```python
from build123d import *

# Parameters (mm, degrees)
FILLET1_R                    = 1.5
CUT_EXTRUDE1_START           = -35
CUT_EXTRUDE1_DEPTH           = 35
FILLET2_R                    = 2
CIRPATTERN1_COUNT            = 6
FILLET2_OF_CIRPATTERN1_R     = 2
FILLET3_R                    = 5
CHAMFER1_SIZE                = 2
CHAMFER3_SIZE                = 1
CUT_EXTRUDE2_REACH           = 152.223
SKETCH3_W                    = 12
SKETCH3_H                    = 35
CHAMFER4_SIZE                = 0.5
CIRPATTERN2_COUNT            = 6
CHAMFER4_OF_CIRPATTERN2_SIZE = 0.5


with BuildPart() as part:
    # Sketch1 → Revolve1 (revolve)
    with BuildSketch(Plane.XY):
        Polygon((20, 80), (30, 80), (30, 50), (77.5, 50), (77.5, 0), (63, 0), (63, 35), (70, 35), (70, 40), (25, 40), (25, 45), (20, 45), align=None)
    revolve(axis=Axis((0, -1292.390356755, 0), (0, 1, 0)))

    # Fillet1
    fillet1_edges = [part.edges().sort_by_distance(p)[0] for p in [
        (-70, 40, 0),
    ]]
    fillet(fillet1_edges, radius=FILLET1_R)

    # Sketch2 → Cut-Extrude1 (cut)
    with BuildSketch(Plane.XZ.offset(CUT_EXTRUDE1_START)):
        with BuildLine():
            Line((-6.125, 68.8), (6.125, 68.8))
            Line((6.125, 68.8), (6.125, 62.701550021))
            ThreePointArc((6.125, 62.701550021), (0, 63), (-6.125, 62.701550021))
            Line((-6.125, 62.701550021), (-6.125, 68.8))
        make_face()
    cut_extrude1 = extrude(amount=CUT_EXTRUDE1_DEPTH, mode=Mode.SUBTRACT)

    # Fillet2
    fillet2_edges = [part.edges().sort_by_distance(p)[0] for p in [
        (6.125, 17.5, 62.701550021),
        (-6.125, 17.5, 62.701550021),
    ]]
    fillet(fillet2_edges, radius=FILLET2_R)

    # CirPattern1: Cut-Extrude1 ×6 about axis
    cirpattern1_axis = Axis((0, 0, 0), (0, 1, 0))
    for i in range(1, CIRPATTERN1_COUNT):
        add(cut_extrude1.rotate(cirpattern1_axis, i * 360 / CIRPATTERN1_COUNT), mode=Mode.SUBTRACT)

    # Fillet2 of CirPattern1
    fillet2_of_cirpattern1_edges = [part.edges().sort_by_distance(p)[0] for p in [
        (57.363635175, 17.5, 26.046369412),
        (51.238635175, 17.5, 36.655180609),
        (51.238635175, 17.5, -36.655180609),
        (57.363635175, 17.5, -26.046369412),
        (-6.125, 17.5, -62.701550021),
        (6.125, 17.5, -62.701550021),
        (-57.363635175, 17.5, -26.046369412),
        (-51.238635175, 17.5, -36.655180609),
        (-51.238635175, 17.5, 36.655180609),
        (-57.363635175, 17.5, 26.046369412),
    ]]
    fillet(fillet2_of_cirpattern1_edges, radius=FILLET2_OF_CIRPATTERN1_R)

    # Fillet3
    fillet3_edges = [part.edges().sort_by_distance(p)[0] for p in [
        (-30, 50, 0),
    ]]
    fillet(fillet3_edges, radius=FILLET3_R)

    # Chamfer1
    chamfer1_edges = [part.edges().sort_by_distance(p)[0] for p in [
        (-77.5, 50, 0),
        (-30, 80, 0),
        (-20, 80, 0),
    ]]
    chamfer(chamfer1_edges, length=CHAMFER1_SIZE)

    # Chamfer3
    chamfer3_edges = [part.edges().sort_by_distance(p)[0] for p in [
        (-25, 40, 0),
        (-20, 45, 0),
    ]]
    chamfer(chamfer3_edges, length=CHAMFER3_SIZE)

    # Sketch3 → Cut-Extrude2 (cut, up to next)
    with BuildSketch(Plane(origin=(23.3, 0, 0), x_dir=(0, 0, -1), z_dir=(1, 0, 0)), mode=Mode.PRIVATE) as cut_extrude2_sk1:
        with Locations((0, 62.5)):
            Rectangle(SKETCH3_W, SKETCH3_H)
    cut_extrude2_tool1 = extrude(cut_extrude2_sk1.sketch, amount=-CUT_EXTRUDE2_REACH, mode=Mode.PRIVATE) & part.part
    add(cut_extrude2_tool1.solids().sort_by_distance((23.3, 62.5, 0))[0], mode=Mode.SUBTRACT)

    # Sketch6 → Cut-Revolve1 (revolve, cut)
    with BuildSketch(Plane.XY, mode=Mode.PRIVATE) as cut_revolve1_sk:
        Polygon((-67.75, 0), (-67.75, 10), (-70.25, 11.443375673), (-70.25, 0), align=None)
    cut_revolve1 = revolve(cut_revolve1_sk.sketch.rotate(Axis((-70.25, -967.908056453, 0), (0, 1, 0)), 90), axis=Axis((-70.25, -967.908056453, 0), (0, 1, 0)), mode=Mode.SUBTRACT)

    # Chamfer4
    chamfer4_edges = [part.edges().sort_by_distance(p)[0] for p in [
        (-70.25, 0, 2.5),
    ]]
    chamfer(chamfer4_edges, length=CHAMFER4_SIZE)

    # CirPattern2: Cut-Revolve1 ×6 about axis
    cirpattern2_axis = Axis((0, 0, 0), (0, 1, 0))
    for i in range(1, CIRPATTERN2_COUNT):
        add(cut_revolve1.rotate(cirpattern2_axis, i * 360 / CIRPATTERN2_COUNT), mode=Mode.SUBTRACT)

    # Chamfer4 of CirPattern2
    chamfer4_of_cirpattern2_edges = [part.edges().sort_by_distance(p)[0] for p in [
        (-32.959936491, 0, 62.088284616),
        (37.290063509, 0, 59.588284616),
        (70.25, 0, -2.5),
        (32.959936491, 0, -62.088284616),
        (-37.290063509, 0, -59.588284616),
    ]]
    chamfer(chamfer4_of_cirpattern2_edges, length=CHAMFER4_OF_CIRPATTERN2_SIZE)


solid = part.part
```
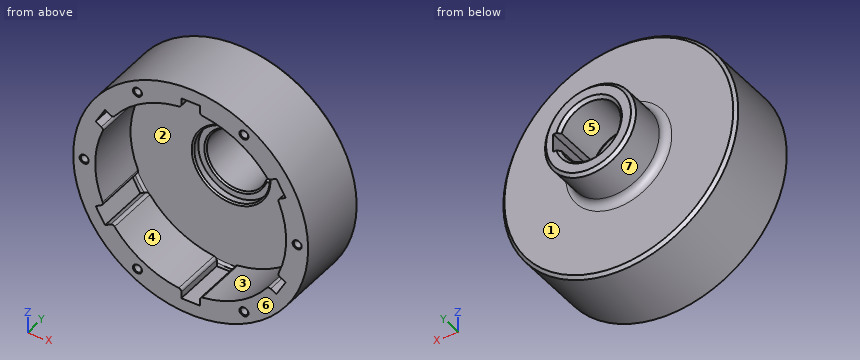
The model under review builds one solid part; all positions refer to its coordinate system, in mm. Face numbers are marked on the shaded views. A direction names the side the tool comes from. Round coordinates to 2 decimals unless told otherwise and drop trailing zeros. Use CSV: the item, a comma, the result in double quotes.
Q1. For pin 1 Ø8 at (x, z) = (-5.5, -49.5) entering from +Y; pin 2 Ø3.5 at (x, y) = (22, 59.5) entering from -Z; pin 3 Ø4.5 at (x, z) = (-35.13, 60.84) entering from -Y, all flat-tipped, find the tip position at first contact; note any pin that passes through.
Checks:
pin 1,"y = 50"
pin 2,"z = -22.13"
pin 3,"y = 10.14"
Q2. To check wall thickness, follow probe 1 along Y at (x, z) = (-30, 59.5); probe 2 along X at (y, z) = (37, 0). State the ranges of each line that lie inside material, in increasing order. Write a range as [from, to].
Checks:
probe 1,"[0, 35], [40, 50]"
probe 2,"[-77.5, -70], [70, 77.5]"
Q3. Consider section A-A (y = 7.5). State how many separate pieces and enclosed holes the cut face has, then the cut area to 3 significant figures.
Checks:
separate pieces,"1"
enclosed holes,"7"
area,"5,840 mm²"
Q4. Mouldability with a two-part tool opening along Z and no side actions: class the marked faces 4, 5, 6 and 7 as released by +Z, released by -Z, zero draft, split by the parting line, or undercut.
Checks:
face 4,"undercut"
face 5,"undercut"
face 6,"zero draft"
face 7,"split by the parting line"
Q5. For the marked faces 1, 2 and 3, list the 3-axis set-ups (+Z, -Z, +X, -X, +Y, -Y) from which the entire face can be reached by the end or side of a thin tool; tool diameter is ignored.
Checks:
face 1,"+Y"
face 2,"none"
face 3,"-Y"
